from build123d import *

# Parameters (mm, degrees)
F0_W     = 10
F0_H     = 17.8
F0_R     = 1
F1_DEPTH = 2
F2_R     = 4.99999


# Not quite as in the source:
# - a fillet or chamfer is up to 0.001 mm smaller than in the source, because OpenCascade refuses the exact size


with BuildPart() as f1:
    # F0 (on Front) → F1 (new body)
    with BuildSketch(Plane.XZ):
        with Locations((5, 8.9)):
            Rectangle(F0_W, F0_H)
        with Locations((5, 5)):
            Circle(F0_R, mode=Mode.SUBTRACT)
        with Locations((5, 12.8)):
            Circle(F0_R, mode=Mode.SUBTRACT)
    extrude(amount=F1_DEPTH)

    # F2 (radius 5 in the source; OpenCascade refuses exactly that, so slightly less here)
    f2_edges = [f1.edges().sort_by_distance(p)[0] for p in [
        (0, -1, 17.8),
        (10, -1, 17.8),
        (0, -1, 0),
    ]]
    fillet(f2_edges, radius=F2_R)


solid = f1.part
Here's how the part is built. I have some questions about the finished solid (model axes, mm). Give positions to 0.01 mm unless a question says otherwise; leave off trailing zeros. Order: outer loops, then holes, each group sorted by start corner. A loop starts at its lowest first (then second) coordinate and runs counter-clockwise, first axis right, second up. Notation, with made-up numbers: (-27.75, -9.75) -> (-14.75, -9.75) arc R21 ccw to (-14.75, -4.75) -> close; hole circle Ø2 at (-28, 89). An arc over 180 degrees is marked (long way). One line per item, written item: value. Start each with the question number.
1. We'd pull the mould along Z, two halves only. Please class faces 1 (the face through (5.46, -0.99, 11.91)), 2 (the face through (1.43, -1.01, 16.3)), 3 (the face through (7, -1, 0)): released by +Z, released by -Z, zero draft, split by the parting line, or undercut.
2. Imagine slicing it at D-D, the plane z = 1.75. List the corners of the cut face in (x, y) for me, plus the area to 3 significant figures.
3. Will this pin go through, and if not, where does the flat tip stop? pin 1 Ø1.6 at (x, z) = (5, 12.8) entering from +Y.
4. Imagine slicing it at A-A, the plane y = -1.2. Count the separate pieces of the cut face and the enclosed holes in it, plus the area to 3 significant figures.
5. Imagine slicing it at B-B, the plane z = 12.5. List the corners of the cut face in (x, y) for me, plus the area to 3 significant figures.
6. I need wall thicknesses on probe 1 along Z at (x, y) = (5, -1); probe 2 along X at (y, z) = (-1.8, 12.75); probe 3 along X at (y, z) = (-0.9, 4.5). Which ranges of each line are inside material? Lowest first, please. Write a range as from..to.
7. Imagine slicing it at C-C, the plane x = 1. List the corners of the cut face in (y, z) for me.
Values follow:
1. face 1: undercut
1. face 2: released by +Z
1. face 3: released by -Z
2. outline: (1.2, -2) -> (10, -2) -> (10, 0) -> (1.2, 0) -> close
2. area: 17.6 mm2
3. pin 1: passes through
4. separate pieces: 1
4. enclosed holes: 2
4. area: 156 mm2
5. outline: (0, -2) -> (4.05, -2) -> (4.05, 0) -> (0, 0) -> close; (5.95, -2) -> (10, -2) -> (10, 0) -> (5.95, 0) -> close
5. area: 16.2 mm2
6. probe 1: z = 0..4, 6..11.8, 13.8..17.8
6. probe 2: x = 0..4, 6..10
6. probe 3: x = 0.03..4.13, 5.87..10
7. outline: (-2, 2) -> (0, 2) -> (0, 15.8) -> (-2, 15.8) -> close
